from build123d import *

# Parameters (mm, degrees)
SKETCH1_R           = 14.0335
SKETCH1_R_2         = 2.38125
BOSS_EXTRUDE1_DEPTH = 4.7625
CUT_EXTRUDE1_DEPTH  = 219.425881909


with BuildPart() as part:
    # Sketch1 → Boss-Extrude1 (new body)
    with BuildSketch(Plane.XY):
        with BuildLine():
            Line((165.542350471, -12.850928795), (158.864493489, -11.70515089))
            ThreePointArc((158.864493489, -11.70515089), (154.154566121, -10.06953751), (150.224583517, -7.001332225))
            ThreePointArc((150.224583517, -7.001332225), (146.294597206, -3.933124046), (141.584665397, -2.297509122))
            Line((141.584665397, -2.297509122), (-187.944818486, 54.242725653))
            ThreePointArc((-187.944818486, 54.242725653), (-189.457270687, 55.108983561), (-190.055285337, 56.746143572))
            Line((-190.055285337, 56.746143572), (-190.055285337, 107.546143572))
            Line((-190.055285337, 107.546143572), (128.771239178, 52.842308466))
            ThreePointArc((128.771239178, 52.842308466), (139.104704977, 55.649471309), (143.618904922, 65.359398058))
            Line((143.618904922, 65.359398058), (143.618904922, 107.546143572))
            Line((143.618904922, 107.546143572), (189.37285399, 107.546143572))
            Line((189.37285399, 107.546143572), (189.37285399, 7.239))
            ThreePointArc((189.37285399, 7.239), (182.127563077, -8.345432433), (165.542350471, -12.850928795))
        make_face()
        with Locations(Location((168.98935399, 7.239, 0), (0, 0, 180))):
            Circle(SKETCH1_R, mode=Mode.SUBTRACT)
        with Locations(Location((104.970773751, 44.478080628, 0), (0, 0, 180))):
            Circle(SKETCH1_R_2, mode=Mode.SUBTRACT)
        with Locations(Location((79.936594567, 48.773412116, 0), (0, 0, 180))):
            Circle(SKETCH1_R_2, mode=Mode.SUBTRACT)
        with Locations(Location((54.902415383, 53.068743605, 0), (0, 0, 180))):
            Circle(SKETCH1_R_2, mode=Mode.SUBTRACT)
        with Locations(Location((29.868236199, 57.364075093, 0), (0, 0, 180))):
            Circle(SKETCH1_R_2, mode=Mode.SUBTRACT)
        with Locations(Location((4.834057015, 61.659406581, 0), (0, 0, 180))):
            Circle(SKETCH1_R_2, mode=Mode.SUBTRACT)
        with Locations(Location((-20.200122168, 65.95473807, 0), (0, 0, 180))):
            Circle(SKETCH1_R_2, mode=Mode.SUBTRACT)
        with Locations(Location((-45.234301352, 70.250069558, 0), (0, 0, 180))):
            Circle(SKETCH1_R_2, mode=Mode.SUBTRACT)
        with Locations(Location((-70.268480536, 74.545401047, 0), (0, 0, 180))):
            Circle(SKETCH1_R_2, mode=Mode.SUBTRACT)
        with Locations(Location((-170.405197271, 91.726727, 0), (0, 0, 180))):
            Circle(SKETCH1_R_2, mode=Mode.SUBTRACT)
        with Locations(Location((-145.371018087, 87.431395512, 0), (0, 0, 180))):
            Circle(SKETCH1_R_2, mode=Mode.SUBTRACT)
        with Locations(Location((-120.336838903, 83.136064023, 0), (0, 0, 180))):
            Circle(SKETCH1_R_2, mode=Mode.SUBTRACT)
        with Locations(Location((-95.30265972, 78.840732535, 0), (0, 0, 180))):
            Circle(SKETCH1_R_2, mode=Mode.SUBTRACT)
    extrude(amount=BOSS_EXTRUDE1_DEPTH)

    # Sketch3 → Cut-Extrude1 (cut, through all)
    with BuildSketch(Plane.XY.offset(4.7625)):
        with BuildLine():
            Line((125.87285399, 333.30748602), (115.993328583, 323.427960612))
            ThreePointArc((115.993328583, 323.427960612), (112.023332702, 320.973988275), (107.375068785, 320.553881036))
            Line((107.375068785, 320.553881036), (17.92285399, 333.30748602))
            Line((17.92285399, 333.30748602), (125.87285399, 333.30748602))
        make_face()
    extrude(amount=-CUT_EXTRUDE1_DEPTH, mode=Mode.SUBTRACT)


solid = part.part
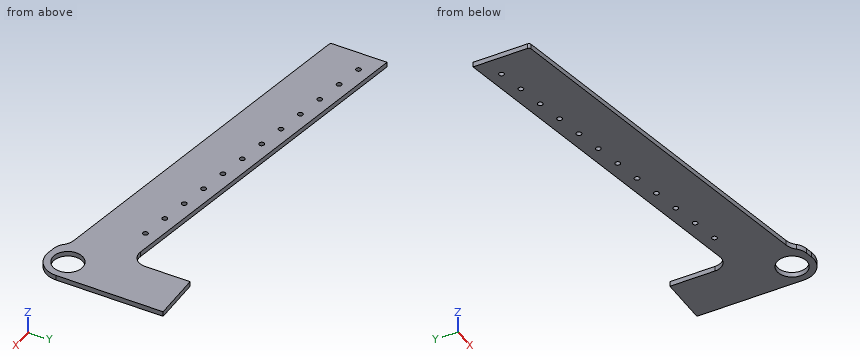
Model file for the job. Use its own axes, mm. Coordinates: 2 decimals unless noted, no trailing zeros. Loops run counter-clockwise (first coordinate to the right, second up) from the corner with the lowest first, then second, coordinate; pieces in that order, holes last. Notation, with made-up numbers: (-29.5, -2.5) -> (-10.5, -2.5) arc R18 ccw to (-10.5, 24.5) -> close; hole circle Ø8 at (33.5, -23). An arc over 180 degrees is marked (long way). Use one line per item in the form item = value. Start each with the question number.
(1) Cut at D-D on x = -104. Give the cut face in (y, z), and give its area (3 significant figures).
(2) Cut at B-B on z = 3.3. Give the number of separate pieces and of enclosed holes in the cut face, and give its area (3 significant figures).
(3) Cut at C-C on y = 2. Give the cut face in (x, z), and give its area (3 significant figures).
(4) Cut at A-A on y = 16.5. Give the cut face in (x, z).
(5) Probe probe 1 along Y at (x, z) = (106, 0.5); probe 2 along Y at (x, z) = (-175, 2.4); probe 3 along Y at (x, z) = (-135, 2.95). List the from-to ranges inside material, lowest first. Write a range as from..to.
(6) Flat gauge pins, fed straight in: pin 1 (1.5 mm diameter, centred on x = -53.5, z = 0.5, fed in from -Y); pin 2 (5.5 mm diameter, centred on x = -95.3, y = 78.84, fed in from -Z); pin 3 (2 mm diameter, centred on x = 8, z = 0.5, fed in from -Y); pin 4 (2 mm diameter, centred on x = -142.5, z = 1.5, fed in from +Y). Where does each tip first touch, or does it go through?
Values:
q1.outline = (39.84, 0) -> (92.78, 0) -> (92.78, 4.76) -> (39.84, 4.76) -> close
q1.area = 252 mm2
q2.separate_pieces = 1
q2.enclosed_holes = 13
q2.area = 22,200 mm2
q3.outline = (116.54, 0) -> (155.97, 0) -> (155.97, 4.76) -> (116.54, 4.76) -> close; (182.01, 0) -> (188.69, 0) -> (188.69, 4.76) -> (182.01, 4.76) -> close
q3.area = 220 mm2
q4.outline = (32.03, 0) -> (158.45, 0) -> (158.45, 4.76) -> (32.03, 4.76) -> close; (179.53, 0) -> (189.37, 0) -> (189.37, 4.76) -> (179.53, 4.76) -> close
q5.probe_1 = 3.81..42.33, 46.63..56.75
q5.probe_2 = 52.02..104.96
q5.probe_3 = 45.16..98.1
q6.pin_1 = 31.05
q6.pin_2 = 0
q6.pin_3 = 20.45
q6.pin_4 = 99.56
